Build history of the part. All positions in model axes, mm. Round coordinates to 2 decimals unless told otherwise and drop trailing zeros. Write each loop counter-clockwise with the first axis right and the second up, starting at its lowest first coordinate (ties: lowest second). Pieces come first, ordered by that corner, then holes.
1) Saw through at A-A (z = 0). Write the cut outline in (x, y), plus the area to 3 significant figures.
2) Saw through at D-D (x = -25.4). Write the cut outline in (y, z), plus the area to 3 significant figures.
3) Wall check: probe 1 along X at (y, z) = (0.95, -25.4); probe 2 along X at (y, z) = (-0.25, 0). Give the ranges that are in metal, low to high.
4) Saw through at B-B (x = 0). Write the cut outline in (y, z).
5) Saw through at C-C (z = -25.4). Write the cut outline in (x, y), plus the area to 3 significant figures.
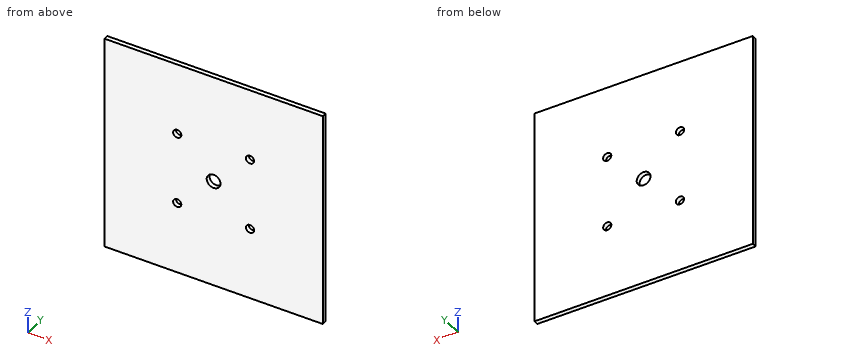
from build123d import *

# Parameters (mm, degrees)
SKETCH1_W           = 152.4
SKETCH1_H           = 3.175
BOSS_EXTRUDE1_DEPTH = 76.2
SKETCH2_R           = 2.8575
SKETCH2_R_2         = 4.826
CUT_EXTRUDE1_DEPTH  = 4.175


with BuildPart() as part:
    # Sketch1 → Boss-Extrude1 (new body, symmetric)
    with BuildSketch(Plane.XY):
        Rectangle(SKETCH1_W, SKETCH1_H)
    extrude(amount=BOSS_EXTRUDE1_DEPTH, both=True)

    # Sketch2 → Cut-Extrude1 (cut, through all)
    with BuildSketch(Plane(origin=(0, 1.5875, 0), x_dir=(1, 0, 0), z_dir=(0, 1, 0))):
        with Locations((-25.4, 25.4)):
            Circle(SKETCH2_R)
        with Locations((25.4, 25.4)):
            Circle(SKETCH2_R)
        with Locations((25.4, -25.4)):
            Circle(SKETCH2_R)
        with Locations((-25.4, -25.4)):
            Circle(SKETCH2_R)
        Circle(SKETCH2_R_2)
    extrude(amount=-CUT_EXTRUDE1_DEPTH, mode=Mode.SUBTRACT)


solid = part.part
Evaluation:
1. outline: (-76.2, -1.59) - (-4.83, -1.59) - (-4.83, 1.59) - (-76.2, 1.59) - close; (4.83, -1.59) - (76.2, -1.59) - (76.2, 1.59) - (4.83, 1.59) - close
1. area: 453 mm2
2. outline: (-1.59, -76.2) - (1.59, -76.2) - (1.59, -28.26) - (-1.59, -28.26) - close; (-1.59, -22.54) - (1.59, -22.54) - (1.59, 22.54) - (-1.59, 22.54) - close; (-1.59, 28.26) - (1.59, 28.26) - (1.59, 76.2) - (-1.59, 76.2) - close
2. area: 448 mm2
3. probe 1: x = -76.2 to -28.26, -22.54 to 22.54, 28.26 to 76.2
3. probe 2: x = -76.2 to -4.83, 4.83 to 76.2
4. outline: (-1.59, -76.2) - (1.59, -76.2) - (1.59, -4.83) - (-1.59, -4.83) - close; (-1.59, 4.83) - (1.59, 4.83) - (1.59, 76.2) - (-1.59, 76.2) - close
5. outline: (-76.2, -1.59) - (-28.26, -1.59) - (-28.26, 1.59) - (-76.2, 1.59) - close; (-22.54, -1.59) - (22.54, -1.59) - (22.54, 1.59) - (-22.54, 1.59) - close; (28.26, -1.59) - (76.2, -1.59) - (76.2, 1.59) - (28.26, 1.59) - close
5. area: 448 mm2
